from build123d import *

# Parameters (mm, degrees)
SKETCH1_R           = 8.275
BOSS_EXTRUDE1_DEPTH = 61.25
CUT_EXTRUDE1_START  = -7.75
SKETCH2_R           = 8.275
SKETCH2_R_2         = 6.5
SKETCH2_R_3         = 4.75
CUT_EXTRUDE1_DEPTH  = 7.75
CUT_EXTRUDE3_START  = -51.5
SKETCH3_R           = 4.75
CUT_EXTRUDE3_DEPTH  = 51.5


with BuildPart() as part:
    # Sketch1 → Boss-Extrude1 (new body)
    with BuildSketch(Plane(origin=(0, 0, 0), x_dir=(1, 0, 0), z_dir=(0, 1, 0))):
        with Locations(Location((0, 0, 0), (0, 0, 270))):
            Circle(SKETCH1_R)
    extrude(amount=BOSS_EXTRUDE1_DEPTH)

    # Sketch2 → Cut-Extrude1 (cut)
    # profile 1 of 2: a face of its own
    with BuildSketch(Plane(origin=(0, 61.25, 0), x_dir=(1, 0, 0), z_dir=(0, 1, 0)).offset(CUT_EXTRUDE1_START)):
        with Locations(Location((0, 0, 0), (0, 0, 270))):
            Circle(SKETCH2_R)
        with Locations(Location((0, 0, 0), (0, 0, 270))):
            Circle(SKETCH2_R_2, mode=Mode.SUBTRACT)
    # profile 2 of 2: a face of its own
    with BuildSketch(Plane(origin=(0, 61.25, 0), x_dir=(1, 0, 0), z_dir=(0, 1, 0)).offset(CUT_EXTRUDE1_START)):
        with Locations(Location((0, 0, 0), (0, 0, 270))):
            Circle(SKETCH2_R_3)
    extrude(amount=CUT_EXTRUDE1_DEPTH, mode=Mode.SUBTRACT)

    # Sketch3 → Cut-Extrude3 (cut)
    with BuildSketch(Plane(origin=(0, 53.5, 0), x_dir=(1, 0, 0), z_dir=(0, 1, 0)).offset(CUT_EXTRUDE3_START)):
        with Locations(Location((0, 0, 0), (0, 0, 270))):
            Circle(SKETCH3_R)
    extrude(amount=CUT_EXTRUDE3_DEPTH, mode=Mode.SUBTRACT)


solid = part.part
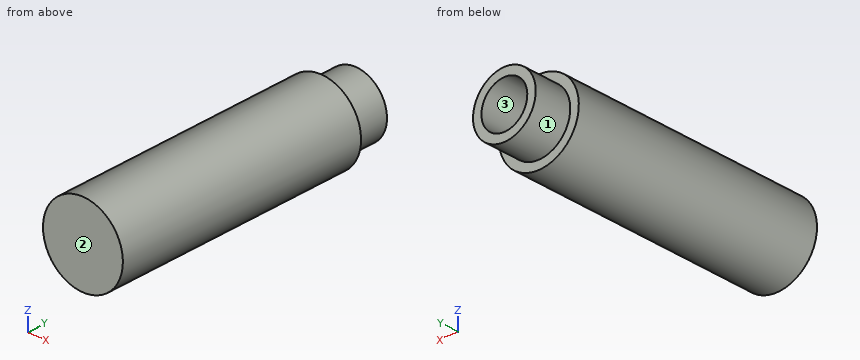
Input: part model. Units: mm. Frame: model coordinates. Face numbers are marked on the shaded views. Give positions to 0.01 mm unless a question says otherwise; leave off trailing zeros. Write each loop counter-clockwise with the first axis right and the second up, starting at its lowest first coordinate (ties: lowest second). Pieces come first, ordered by that corner, then holes.
Q1. First-contact query: P1, Ø4, axis at y = 21.5, z = -6, coming from the +X side; P2, Ø1, axis at x = -3.5, y = 36, coming from the -Z side; P3, Ø1, axis at x = 4, y = 23.5, coming from the +Z side. Flat tips, straight axial feed; report the tip coordinate or a pass-through.
Q2. Section B-B, the plane x = 0. Output: boundary loops of the cut face in (y, z) (3 decimals).
Q3. Material intervals for probe 1 along X at (y, z) = (27, 0) (3 decimals); probe 2 along Z at (x, y) = (1.25, 57); probe 3 along X at (y, z) = (26, 3), sorted ascending.
Q4. Section C-C, the plane y = 45.5. Output: boundary loops of the cut face in (x, z) (3 decimals).
Q5. Pull-direction query (Z, two-part tool) for the marked faces 1, 2 and 3; classes: pulls with the +Z half, pulls with the -Z half, needs draft (parallel to the pull), parting line crosses it, or undercut.
Q6. Section D-D, the plane z = 5.75. Output: boundary loops of the cut face in (x, y), plus the area to 3 significant figures.
Q7. Section A-A, the plane z = 0. Output: boundary loops of the cut face in (x, y) (3 decimals), plus the area to 3 significant figures.
Filled in:
1. P1: stops at x = 7.24
1. P2: stops at z = -7.71
1. P3: stops at z = 7.5
2. outline: (0, -8.275) - (53.5, -8.275) - (53.5, -6.5) - (61.25, -6.5) - (61.25, -4.75) - (2, -4.75) - (2, 4.75) - (61.25, 4.75) - (61.25, 6.5) - (53.5, 6.5) - (53.5, 8.275) - (0, 8.275) - close
3. probe 1: x = -8.275 to -4.75, 4.75 to 8.275
3. probe 2: z = -6.38 to -4.58, 4.58 to 6.38
3. probe 3: x = -7.71 to -3.68, 3.68 to 7.71
4. outline: circle Ø16.55 at (0, 0); hole circle Ø9.5 at (0, 0)
5. face 1: parting line crosses it
5. face 2: needs draft
5. face 3: undercut
6. outline: (-5.95, 0) - (5.95, 0) - (5.95, 53.5) - (3.03, 53.5) - (3.03, 61.25) - (-3.03, 61.25) - (-3.03, 53.5) - (-5.95, 53.5) - close
6. area: 684 mm2
7. outline: (-8.275, 0) - (8.275, 0) - (8.275, 53.5) - (6.5, 53.5) - (6.5, 61.25) - (4.75, 61.25) - (4.75, 2) - (-4.75, 2) - (-4.75, 61.25) - (-6.5, 61.25) - (-6.5, 53.5) - (-8.275, 53.5) - close
7. area: 423 mm2
